from build123d import *

# Parameters (mm, degrees)
F0_W     = 30
F0_H     = 8
F1_DEPTH = 0.6


# Not quite as in the source:
# - a pattern or mirror of a feature is missing from the dataset's text; its kind, count and spacing are read off the source's solid


with BuildPart() as f1:
    # F0 (on Top) → F1 (new body)
    with BuildSketch(Plane.XY):
        Rectangle(F0_W, F0_H)
    extrude(amount=F1_DEPTH)

    # F2 (on Front) → F3 (revolve)
    with BuildSketch(Plane.XZ):
        Polygon((-5.5, 0.6), (-7.3, 15.6), (-7.5, 15.6), (-7.5, 0.6), align=None)
    f3 = revolve(axis=Axis((-7.5, 0, 8.1), (0, 0, -1)))

    # F3_copies: F3 across plane
    add(f3.mirror(Plane(origin=(0, 0, 0), x_dir=(0, 0, 1), z_dir=(1, 0, 0))))


solid = f1.part
For this review, take the finished solid that the model builds, in its own axes (mm). Round coordinates to 2 decimals unless told otherwise and drop trailing zeros. Write each loop counter-clockwise with the first axis right and the second up, starting at its lowest first coordinate (ties: lowest second). Pieces come first, ordered by that corner, then holes. Notation, with made-up numbers: (68.5, -1) - (87.5, -1) arc R10 ccw to (87.5, 5) - close; hole circle Ø5 at (19, 30). An arc over 180 degrees is marked (long way). Use a Markdown table: item, result.
Q1. We need section A-A (z = 1.5). Give the boundary of the cut face in (x, y).
Derived:
| item | result |
|---|---|
| outline | circle Ø3.78 at (-7.5, 0); circle Ø3.78 at (7.5, 0) |
Q2. We need section C-C (z = 13.5). Give the boundary of the cut face in (x, y), plus the area to 3 significant figures.
Derived:
| item | result |
|---|---|
| outline | circle Ø0.9 at (-7.5, 0); circle Ø0.9 at (7.5, 0) |
| area | 1.28 mm2 |
Q3. Wall thickness on line 1 along Z through (x, y) = (-9, 1.5); line 2 along X through (y, z) = (1.5, 3); line 3 along X through (y, z) = (0, 8.25): over which ranges is each line inside the solid? List them lowest first.
Derived:
| item | result |
|---|---|
| line 1 | z = 0 to 0.6 |
| line 2 | x = -8.33 to -6.67, 6.67 to 8.33 |
| line 3 | x = -8.58 to -6.42, 6.42 to 8.58 |
Q4. The part is to be moulded in two halves that separate along X. For faces 1 (the flat face through (0, 0, 0)), 2 (the flat face through (0, 0, 0.6)), say which applies: pulls with the +X half, pulls with the -X half, needs draft (parallel to the pull), parting line crosses it, or undercut.
Derived:
| item | result |
|---|---|
| face 1 | needs draft |
| face 2 | undercut |
Q5. We need section B-B (x = 4.75). Give the boundary of the cut face in (y, z), plus the area to 3 significant figures.
Derived:
| item | result |
|---|---|
| outline | (-4, 0) - (4, 0) - (4, 0.6) - (-4, 0.6) - close |
| area | 4.80 mm2 |
Q6. Clearance check with flat-ended pins moving along their axes: pin 1 (6 mm diameter, centred on x = -4, z = 2, fed in from -Y); pin 2 (4 mm diameter, centred on x = 6, z = 12.5, fed in from -Y); pin 3 (2 mm diameter, centred on y = 1, z = 3, fed in from +X); pin 4 (2 mm diameter, centred on x = 8.5, z = 2.5, fed in from -Y). State where each tip first meets the part, or that it passes through.
Derived:
| item | result |
|---|---|
| pin 1 | stops at y = -4 |
| pin 2 | stops at y = -0.74 |
| pin 3 | stops at x = 9.27 |
| pin 4 | stops at y = -1.83 |
